from build123d import *

# Parameters (mm, degrees)
F0_R      = 2.475
F1_DEPTH  = 2
F2_R      = 3
F3_DEPTH  = 2
F4_R      = 1.99999
F5_W      = 6.8
F5_H      = 8
F5_R      = 2.475
F6_DEPTH  = 3
F7_W      = 4.8
F7_H      = 8
F8_DEPTH  = 3
F9_W      = 2
F9_H      = 6
F10_DEPTH = 2.2
F11_W     = 0.75
F11_H     = 6
F11_W_2   = 2
F12_DEPTH = 2
F13_R     = 1.5


# Not quite as in the source:
# - a fillet or chamfer is up to 0.001 mm smaller than in the source, because OpenCascade refuses the exact size


with BuildPart() as f1:
    # F0 (on Front) → F1 (new body)
    with BuildSketch(Plane.XZ):
        Circle(F0_R)
    extrude(amount=F1_DEPTH)

    # F2 (on face) → F3 (join)
    with BuildSketch(Plane.XZ.offset(2)):
        Circle(F2_R)
    extrude(amount=F3_DEPTH)

    # F4 (radius 2 in the source; OpenCascade refuses exactly that, so slightly less here)
    f4_edges = [f1.edges().sort_by_distance(p)[0] for p in [
        (-3, -4, 0),
    ]]
    fillet(f4_edges, radius=F4_R)

    # F5 (on face) → F6 (join)
    with BuildSketch(Plane(origin=(0, 0, 0), x_dir=(-1, 0, 0), z_dir=(0, 1, 0))):
        Rectangle(F5_W, F5_H)
        Circle(F5_R, mode=Mode.SUBTRACT)
        Circle(F5_R)
    extrude(amount=F6_DEPTH)

    # F7 (on face) → F8 (join)
    with BuildSketch(Plane(origin=(0, 3, 0), x_dir=(-1, 0, 0), z_dir=(0, 1, 0))):
        Rectangle(F7_W, F7_H)
    extrude(amount=F8_DEPTH)

    # F9 (on face) → F10 (join)
    with BuildSketch(Plane(origin=(0, 6, 0), x_dir=(-1, 0, 0), z_dir=(0, 1, 0))):
        Rectangle(F9_W, F9_H)
    extrude(amount=F10_DEPTH)

    # F11 (on face) → F12 (join)
    with BuildSketch(Plane(origin=(0, 8.2, 0), x_dir=(-1, 0, 0), z_dir=(0, 1, 0))):
        with Locations((-1.375, 0)):
            Rectangle(F11_W, F11_H)
        Rectangle(F11_W_2, F11_H)
        with Locations((1.375, 0)):
            Rectangle(F11_W, F11_H)
    extrude(amount=F12_DEPTH)

    # F13
    f13_edges = [f1.edges().sort_by_distance(p)[0] for p in [
        (1.75, 10.2, 0),
        (-1.75, 10.2, 0),
    ]]
    fillet(f13_edges, radius=F13_R)


solid = f1.part
Geometry: final body of the model. Coordinates: model frame, mm. A direction names the side the tool comes from. Round coordinates to 2 decimals unless told otherwise and drop trailing zeros. Loops run counter-clockwise (first coordinate to the right, second up) from the corner with the lowest first, then second, coordinate; pieces in that order, holes last.
Q1. Pull-direction query (Y, two-part tool) for faces 5 (the flat face through (-2, -2, 2)), 6 (the flat face through (1, 7, 0)), 7 (the flat face through (0, 3, -4)), 8 (the flat face through (0, -4, 0)); classes: released by +Y, released by -Y, zero draft, split by the parting line, or undercut.
Q2. Section B-B on y = -1.75. Return loops of the section in (x, z) (3 decimals).
Q3. Access query for faces 1 (the flat face through (0, 8, 3)), 2 (the flat face through (-1, 7, 0)), 3 (the cylindrical face through (2.36, -0.99, 0.74)), 4 (the flat face through (0, 8, -3)). Directions: +Z, -Z, +X, -X, +Y, -Y. A direction counts if a zero-diameter tool reaches every point of the face in a straight line with its end or side. Return the directions, or none.
Q4. Section A-A on y = 4.25. Return loops of the section in (x, z), plus the area to 3 significant figures.
Q5. Material intervals for L1, parallel to X at y = 4.75, z = 2.5; L2, parallel to Y at x = 1.5, z = -0.75; L3, parallel to Y at x = 3.25, z = -1.5, sorted ascending.
Q6. Pin query (flat end, axial travel): P1, Ø0.7, axis at y = 7, z = 0.5, coming from the +X side; P2, Ø0.8, axis at x = -2.5, z = 1.5, coming from the +Y side; P3, Ø0.6, axis at x = -1.5, z = -1, coming from the -Y side. Return the tip coordinate at first contact, or that it passes through.
Evaluation:
1. face 5: undercut
1. face 6: undercut
1. face 7: zero draft
1. face 8: released by -Y
2. outline: circle Ø4.95 at (0, 0)
3. face 1: +Z, +X, -X, +Y
3. face 2: +Z, -Z, -X
3. face 3: none
3. face 4: -Z, +X, -X, +Y
4. outline: (-2.4, -4) - (2.4, -4) - (2.4, 4) - (-2.4, 4) - close
4. area: 38.4 mm2
5. L1: x = -2.4 to 2.4
5. L2: y = -3.88 to 6, 8.2 to 9.53
5. L3: y = 0 to 3
6. P1: stops at x = 1
6. P2: stops at y = 6
6. P3: stops at y = -3.94
